Verification items for the finished model (mm, model axes). A direction names the side the tool comes from. Round coordinates to 2 decimals unless told otherwise and drop trailing zeros. Loops run counter-clockwise (first coordinate to the right, second up) from the corner with the lowest first, then second, coordinate; pieces in that order, holes last. Notation, with made-up numbers: (67.5, -3.75) - (105.5, -3.75) arc R25 cw to (105.5, 17.25) - close; hole circle Ø9 at (37, 4.5). An arc over 180 degrees is marked (long way). Use a Markdown table: item, result. Add a question column.
Autodesk Inventor part; units mm, degrees
ref_plane "YZ Plane" through (0, 0, 0) normal (1, 0, 0) x (0, 1, 0)
ref_plane "XZ Plane" through (0, 0, 0) normal (0, 1, 0) x (-1, 0, 0)
ref_plane "XY Plane" through (0, 0, 0) normal (0, 0, 1) x (1, 0, 0)
sketch "Sketch1" plane through (0, 0, 0) normal (1, 0, 0) x (0, 1, 0)
  line L0 (25.4, 25.4) -> (0, 25.4) construction
  line L1 (0, 25.4) -> (0, 0)
  line L2 (0, 0) -> (25.4, 0)
  line L3 (25.4, 0) -> (25.4, 25.4) construction
  line L4 (25.4, 25.4) -> (3.175, 25.4) construction
  line L5 (3.175, 25.4) -> (3.175, 3.175)
  line L6 (3.175, 3.175) -> (25.4, 3.175)
  line L7 (25.4, 3.175) -> (25.4, 25.4) construction
  line L8 (25.4, 3.175) -> (25.4, 0)
  line L9 (3.175, 25.4) -> (0, 25.4)
  point P0 (0, 0)
  dimension "d1" = 25.4
  dimension "d2" = 3.175
extrude "Extrusion1" add sketch "Sketch1" along normal mid plane 390.8
sketch "Sketch2" plane through (-195.4, 3.175, 25.4) normal (0, 1, 0) x (1, 0, 0)
  line L0 (0, 0) -> (390.8, 0)
  line L1 (0, 0) -> (29.575, 0)
  line L2 (29.575, 0) -> (29.575, 22.225)
  line L3 (29.575, 22.225) -> (0, 22.225)
  line L4 (0, 22.225) -> (0, 0)
  line L5 (0, 22.225) -> (390.8, 22.225)
  point P0 (195.4, 25.4)
  point P1 (29.575, 0)
  dimension "d5" = 29.575
extrude "Extrusion2" cut sketch "Sketch2" against normal blind 3.175
sketch "Sketch3" plane through (-195.4, 25.4, 3.175) normal (0, 0, 1) x (1, 0, 0)
  line L0 (0, 0) -> (390.8, 0) construction
  line L1 (0, 0) -> (25.4, 0) construction
  line L2 (25.4, 0) -> (25.4, -25.4) construction
  line L3 (25.4, -25.4) -> (0, -25.4) construction
  line L4 (0, -25.4) -> (0, 0) construction
  line L5 (3.175, 0) -> (22.225, 0) construction
  line L6 (22.225, 0) -> (22.225, -25.4) construction
  line L7 (22.225, -25.4) -> (3.175, -25.4) construction
  line L8 (3.175, -25.4) -> (3.175, 0) construction
  line L9 (8.4667, -8.4667) -> (16.9333, -8.4667) construction
  line L10 (16.9333, -8.4667) -> (16.9333, -16.9333) construction
  line L11 (16.9333, -16.9333) -> (8.4667, -16.9333) construction
  line L12 (8.4667, -16.9333) -> (8.4667, -8.4667) construction
  circle A0 centre (8.4667, -8.4667) radius 2.4257
  circle A1 centre (16.9333, -16.9333) radius 2.4257
  point P0 (195.4, -25.4)
  point P1 (12.7, 0)
  point P2 (12.7, 0)
  point P3 (16.9333, -12.7)
  point P4 (22.225, -12.7)
  point P5 (12.7, -8.4667)
  dimension "d8" = 25.4
  dimension "d9" = 3.175
  dimension "d10" = 4.8514
  dimension "d11" = 8.4667
extrude "Extrusion3" cut sketch "Sketch3" against normal blind 3.175
mirror "Mirror1" about plane through (0, 0, 0) normal (1, 0, 0) of "Extrusion2", "Extrusion3"
properties part number "beamZ"
Q1. Section check A-A on x = -89.5. Record the cut outline in (y, z) (3 decimals), plus the area to 3 significant figures.
Q2. Thickness scan on line 1 along Z through (x, y) = (-136, 12.75) (3 decimals). Record the ranges inside material, lowest first.
Q3. Section check B-B on z = 19. Record the cut outline in (x, y) (3 decimals), plus the area to 3 significant figures.
Q4. Set-up check for faces 1 (the face through (-2, 3.175, 14)), 2 (the face through (-3, 13, 0)): record each of +Z, -Z, +X, -X, +Y, -Y from which the full face is reachable in a straight line by a thin tool's end or side.
Q5. Go/stop test with flat-tipped pins: pin 1 Ø10 at (x, y) = (48, 11) entering from +Z (3 decimals); pin 2 Ø12 at (x, z) = (140.5, 8) entering from +Y; pin 3 Ø1 at (y, z) = (2, 14) entering from +X (3 decimals); pin 4 Ø3.5 at (y, z) = (2, 17.5) entering from -X (3 decimals). Record where each tip stops, or that it passes through.
Determined:
| question | item | result |
|---|---|---|
| 1 | outline | (0, 0) - (25.4, 0) - (25.4, 3.175) - (3.175, 3.175) - (3.175, 25.4) - (0, 25.4) - close |
| 1 | area | 151 mm² |
| 2 | line 1 | z = 0 to 3.175 |
| 3 | outline | (-165.825, 0) - (165.825, 0) - (165.825, 3.175) - (-165.825, 3.175) - close |
| 3 | area | 1,050 mm² |
| 4 | face 1 | +Z, +X, -X, +Y |
| 4 | face 2 | -Z, +X, -X, +Y, -Y |
| 5 | pin 1 | stops at z = 3.175 |
| 5 | pin 2 | stops at y = 25.4 |
| 5 | pin 3 | stops at x = 165.825 |
| 5 | pin 4 | stops at x = -165.825 |
